Geometry: final body of the model. Coordinates: model frame, mm. A direction names the side the tool comes from. Give positions to 0.01 mm unless a question says otherwise; leave off trailing zeros. Write each loop counter-clockwise with the first axis right and the second up, starting at its lowest first coordinate (ties: lowest second). Pieces come first, ordered by that corner, then holes. Notation, with made-up numbers: (-8.5, 6.5) -> (39.5, 6.5) arc R25 cw to (39.5, 19.5) -> close; hole circle Ø10 at (85.25, 81). An arc over 180 degrees is marked (long way). Answer as a JSON object with one key per item and string values. Group by question number.
(1) Material intervals for probe 1 along Y at (x, z) = (0, -3); probe 2 along Z at (x, y) = (5.25, 2.25); probe 3 along Y at (x, z) = (0, 0.5), sorted ascending.
(2) Section query C-C on z = -3. Output: boundary loops of the cut face in (x, y).
(3) Section query A-A on y = 0. Output: boundary loops of the cut face in (x, z).
(4) Section query D-D on y = -2.25. Output: boundary loops of the cut face in (x, z).
(5) Draft query along Z for faces 1 (the face through (-1.08, -4.88, 0.04)), 2 (the face through (-5.158, -3.955, 2.993)), 3 (the face through (-1, 2, -3.5)). Return one class per face: +Z half, -Z half, draft (parallel to the pull), parting line (faces both ways), or undercut.
(6) Set-up query: faces 4 (the face through (1, 2, 3.5)), 5 (the face through (2, -5, 2.5)). Return all of +Z, -Z, +X, -X, +Y, -Y with unobstructed straight access to the full face (end or side cutting, diameter ignored); none if empty.
(7) Contact query for flat-ended pins moving along their axis: pin 1 Ø1 at (y, z) = (-2, 0) entering from -X; pin 2 Ø3 at (x, z) = (-4, 1.5) entering from +Y. Output: stop coordinate, or through.
from build123d import *

# Parameters (mm, degrees)
SKETCH_1_R      = 5
SKETCH_1_R_2    = 2
EXTRUDE_1_DEPTH = 2.5
SKETCH_2_R      = 6.5
SKETCH_2_R_2    = 2
EXTRUDE_2_DEPTH = 1
SKETCH_3_R      = 6.5
SKETCH_3_R_2    = 2
EXTRUDE_3_DEPTH = 1


with BuildPart() as part:
    # 스케치1 → 보스-돌출1 (new body, symmetric)
    with BuildSketch(Plane.XY):
        Circle(SKETCH_1_R)
        Circle(SKETCH_1_R_2, mode=Mode.SUBTRACT)
    extrude(amount=EXTRUDE_1_DEPTH, both=True)

    # 스케치2 → 보스-돌출2 (add)
    with BuildSketch(Plane(origin=(0, 0, -2.5), x_dir=(-1, 0, 0), z_dir=(0, 0, -1))):
        Circle(SKETCH_2_R)
        Circle(SKETCH_2_R_2, mode=Mode.SUBTRACT)
    extrude(amount=EXTRUDE_2_DEPTH)

    # 스케치3 → 보스-돌출3 (add)
    with BuildSketch(Plane.XY.offset(2.5)):
        Circle(SKETCH_3_R)
        Circle(SKETCH_3_R_2, mode=Mode.SUBTRACT)
    extrude(amount=EXTRUDE_3_DEPTH)


solid = part.part
Answer list:
{
 "1": {"probe 1": "-6.5 to -2, 2 to 6.5", "probe 2": "-3.5 to -2.5, 2.5 to 3.5", "probe 3": "-5 to -2, 2 to 5"},
 "2": {"outline": "circle Ø13 at (0, 0); hole circle Ø4 at (0, 0)"},
 "3": {"outline": "(-6.5, -3.5) -> (-2, -3.5) -> (-2, 3.5) -> (-6.5, 3.5) -> (-6.5, 2.5) -> (-5, 2.5) -> (-5, -2.5) -> (-6.5, -2.5) -> close; (2, -3.5) -> (6.5, -3.5) -> (6.5, -2.5) -> (5, -2.5) -> (5, 2.5) -> (6.5, 2.5) -> (6.5, 3.5) -> (2, 3.5) -> close"},
 "4": {"outline": "(-6.1, -3.5) -> (6.1, -3.5) -> (6.1, -2.5) -> (4.47, -2.5) -> (4.47, 2.5) -> (6.1, 2.5) -> (6.1, 3.5) -> (-6.1, 3.5) -> (-6.1, 2.5) -> (-4.47, 2.5) -> (-4.47, -2.5) -> (-6.1, -2.5) -> close"},
 "5": {"face 1": "undercut", "face 2": "draft", "face 3": "-Z half"},
 "6": {"face 4": "+Z, +X, -X, +Y, -Y", "face 5": "none"},
 "7": {"pin 1": "x = -4.77", "pin 2": "y = 5.83"}
}
